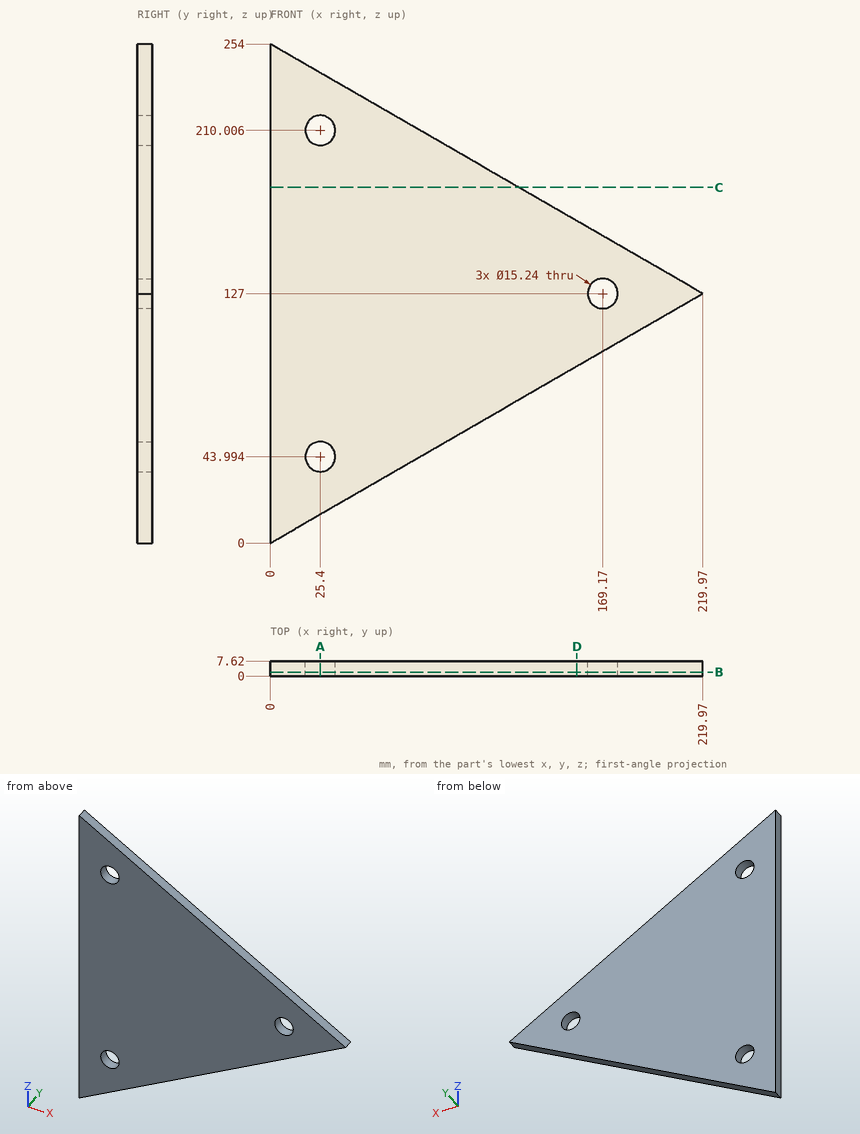
The drawing under review shows one solid part. Ordinate dimensions are in mm from its lowest x, y, z. Coordinates: 2 decimals unless noted, no trailing zeros. Write each loop counter-clockwise with the first axis right and the second up, starting at its lowest first coordinate (ties: lowest second). Pieces come first, ordered by that corner, then holes.
1) To check wall thickness, follow L1, parallel to Z at x = 25.4, y = 5.25 (1 decimal); L2, parallel to X at y = 2.5, z = 55.5 (1 decimal); L3, parallel to X at y = 6.25, z = 219 (1 decimal). State the ranges of each line that lie inside material, in increasing order.
2) Add section A-A (x = 25.4). Write out the cut boundary in (y, z) (1 decimal), plus the area to 3 significant figures.
3) Add section C-C (z = 181). Write out the cut boundary in (x, y).
4) Add section B-B (y = 2). Write out the cut boundary in (x, z) (1 decimal), plus the area to 3 significant figures.
5) Insertion check: pin 1 (3 mm diameter, centred on x = 104, y = 3, fed in from +Z); pin 2 (13.5 mm diameter, centred on x = 25.4, z = 43.99, fed in from -Y); pin 3 (4 mm diameter, centred on x = 80, y = 2, fed in from -Z). Each pin has a flat end and moves straight along its axis. Give the tip position at first contact, or say it passes through.
6) Add section D-D (x = 156). Write out the cut boundary in (y, z), plus the area to 3 significant figures.
Check result:
1. L1: z = 14.7 to 36.4, 51.6 to 202.4, 217.6 to 239.3
1. L2: x = 0 to 96.1
1. L3: x = 0 to 60.6
2. outline: (0, 14.7) - (7.6, 14.7) - (7.6, 36.4) - (0, 36.4) - close; (0, 51.6) - (7.6, 51.6) - (7.6, 202.4) - (0, 202.4) - close; (0, 217.6) - (7.6, 217.6) - (7.6, 239.3) - (0, 239.3) - close
2. area: 1,480 mm2
3. outline: (0, 0) - (126.44, 0) - (126.44, 7.62) - (0, 7.62) - close
4. outline: (0, 0) - (220, 127) - (0, 254) - close; hole circle Ø15.2 at (25.4, 44); hole circle Ø15.2 at (25.4, 210); hole circle Ø15.2 at (169.2, 127)
4. area: 27,400 mm2
5. pin 1: stops at z = 194.82
5. pin 2: passes through
5. pin 3: stops at z = 45.03
6. outline: (0, 90.07) - (7.62, 90.07) - (7.62, 163.93) - (0, 163.93) - close
6. area: 563 mm2
